Design review of the part built by this model. Coordinates are the model's own, in mm. Face numbers are marked on the shaded views. A direction names the side the tool comes from. Give positions to 0.01 mm unless a question says otherwise; leave off trailing zeros. Order: outer loops, then holes, each group sorted by start corner. A loop starts at its lowest first (then second) coordinate and runs counter-clockwise, first axis right, second up. Notation, with made-up numbers: (-4.75, 32.5) -> (34.25, 32.5) arc R18 cw to (34.25, 59.5) -> close; hole circle Ø7 at (20, -18.5). An arc over 180 degrees is marked (long way). One line per item, written item: value. Start each with the question number.
1) Consider section D-D (y = -10). State the section outline as (x, z) points.
2) Wall thickness on line 1 along Y through (x, z) = (-3.5, -4.5); line 2 along X through (y, z) = (-9.5, -3); line 3 along Z through (x, y) = (-5, -0.75): over which ranges is each line inside the solid? List them lowest first. Write a range as from..to.
3) Consider section C-C (x = -6). State the section outline as (y, z) points.
4) Consider section B-B (z = -2.5). State the section outline as (x, y) points, plus the area to 3 significant figures.
5) Tool access review of the marked faces 1 and 2: name each direction out of +Z, -Z, +X, -X, +Y, -Y from which nothing blocks a thin tool from reaching the whole face with its end or side.
6) For pin 1 (3 mm diameter, centred on x = -1, z = -2.5, fed in from +Y); pin 2 (1.8 mm diameter, centred on x = -7.5, z = -5, fed in from +Y); pin 3 (3 mm diameter, centred on x = -3.47, y = -3.53, fed in from +Z); pin 4 (3.5 mm diameter, centred on x = -5, y = -2, fed in from -Z), all flat-tipped, find the tip position at first contact; note any pin that passes through.
7) The part is to be moulded in two halves that separate along Y. For the marked faces 3, 4 and 5, say which applies: released by +Y, released by -Y, zero draft, split by the parting line, or undercut.
from build123d import *

# Parameters (mm, degrees)
F1_DEPTH = 7
F0_R     = 1.25
F2_DEPTH = 6.4


with BuildPart() as f1:
    # F0 (on Top) → F1 (new body)
    with BuildSketch(Plane.XY):
        with BuildLine():
            Line((0.053334, -14.707793), (0.053334, -3.527793))
            ThreePointArc((0.053334, -3.527793), (-1.874686, -6.66722), (-5.546666, -6.367512))
            Line((-5.546666, -6.367512), (-5.546666, -11.457793))
            Line((-5.546666, -11.457793), (-7.846666, -11.457793))
            Line((-7.846666, -11.457793), (-7.846666, -14.707793))
            Line((-7.846666, -14.707793), (-3.466666, -14.707793))
            Line((-3.466666, -14.707793), (0.053334, -14.707793))
        make_face()
    extrude(amount=-F1_DEPTH)

    # F0 (on Top) → F2 (join)
    with BuildSketch(Plane.XY):
        with BuildLine():
            ThreePointArc((-5.546666, -6.367512), (-1.874686, -6.66722), (0.053334, -3.527793))
            ThreePointArc((0.053334, -3.527793), (-5.058645, -0.388367), (-5.546666, -6.367512))
        make_face()
        with Locations((-3.466666, -3.527793)):
            Circle(F0_R, mode=Mode.SUBTRACT)
    extrude(amount=-F2_DEPTH)


solid = f1.part
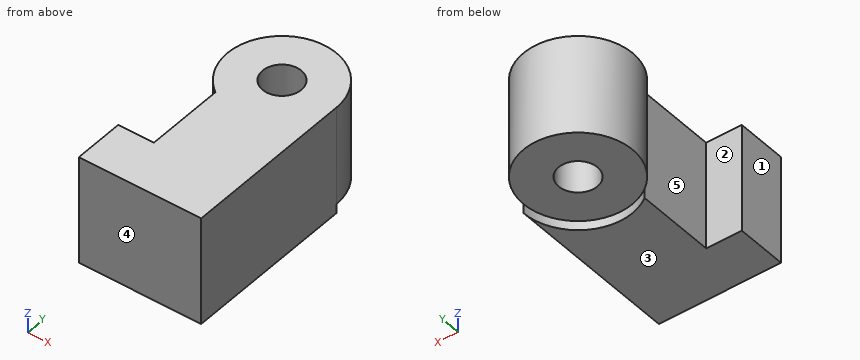
Checked values:
1. outline: (-5.55, -7) -> (0.05, -7) -> (0.05, 0) -> (-5.55, 0) -> close
2. line 1: y = -14.71..-4.78, -2.28..-0.01
2. line 2: x = -5.55..0.05
2. line 3: z = -6.4..0
3. outline: (-14.71, -7) -> (-11.46, -7) -> (-11.46, 0) -> (-14.71, 0) -> close; (-5.97, -6.4) -> (-1.08, -6.4) -> (-1.08, 0) -> (-5.97, 0) -> close
4. outline: (-7.85, -14.71) -> (0.05, -14.71) -> (0.05, -3.53) arc R3.52 ccw (long way) to (-5.55, -6.37) -> (-5.55, -11.46) -> (-7.85, -11.46) -> close; hole circle Ø2.5 at (-3.47, -3.53)
4. area: 87.5 mm^2
5. face 1: +Z, -Z, -X, +Y, -Y
5. face 2: +Z, -Z, -X
6. pin 1: stops at y = -0.14
6. pin 2: stops at y = -1.92
6. pin 3: stops at z = 0
6. pin 4: stops at z = -6.4
7. face 3: zero draft
7. face 4: released by -Y
7. face 5: undercut
